Geometry: final body of the model. Coordinates: model frame, mm. A direction names the side the tool comes from. Give positions to 0.01 mm unless a question says otherwise; leave off trailing zeros. Loops run counter-clockwise (first coordinate to the right, second up) from the corner with the lowest first, then second, coordinate; pieces in that order, holes last.
Autodesk Inventor part; units mm, degrees
ref_plane "YZ Plane" through (0, 0, 0) normal (1, 0, 0) x (0, 1, 0)
ref_plane "XZ Plane" through (0, 0, 0) normal (0, 1, 0) x (-1, 0, 0)
ref_plane "XY Plane" through (0, 0, 0) normal (0, 0, 1) x (1, 0, 0)
sketch "Skizze1" plane through (0, 0, 0) normal (1, 0, 0) x (0, 1, 0)
  line L0 (105.1634, 173.9786) -> (55.1634, 173.9786)
  line L1 (55.1634, 173.9786) -> (55.1634, 93.4786)
  line L2 (55.1634, 93.4786) -> (105.1634, 93.4786)
  line L3 (105.1634, 93.4786) -> (105.1634, 173.9786)
  point P0 (0, 0)
  dimension "d0" = 80.5
  dimension "d1" = 50
extrude "Extrusion1" add sketch "Skizze1" along normal blind 5
sketch "Skizze2" plane through (5, 0, 0) normal (1, 0, 0) x (0, 0, -1)
  line L0 (-173.9786, 105.1639) -> (-168.9786, 105.1634)
  line L1 (-93.4786, 105.1634) -> (-173.9786, 105.1634)
  line L2 (-173.9786, 55.1634) -> (-93.4786, 55.1634)
  line L3 (-168.9786, 55.1634) -> (-173.9786, 55.1634)
  line L4 (-173.9786, 55.1634) -> (-173.9786, 105.1639)
  line L5 (-168.9786, 105.1634) -> (-168.9786, 55.1634)
  line L6 (-93.4786, 105.1634) -> (-98.4786, 105.1634)
  line L7 (-98.4786, 55.1634) -> (-93.4786, 55.1634)
  line L8 (-93.4786, 55.1634) -> (-93.4786, 105.1634)
  line L9 (-93.4786, 105.1634) -> (-98.4786, 105.1634)
  line L10 (-98.4786, 55.1634) -> (-98.4786, 105.1634)
  line L11 (-98.4786, 105.1634) -> (-93.4786, 105.1634)
  line L12 (-93.4786, 55.1634) -> (-98.4786, 55.1634)
  line L13 (-98.4786, 105.1634) -> (-93.4786, 105.1634)
  line L14 (-93.4786, 55.1634) -> (-98.4786, 55.1634)
  line L15 (-98.4786, 105.1634) -> (-93.4786, 105.1634)
  point P0 (0, 0)
  dimension "d4" = 5
  dimension "d5" = 5
extrude "Extrusion2" add sketch "Skizze2" along normal blind 70 contours L1 L8 L2 L10
sketch "Skizze3" plane through (5, 55.1634, 98.4786) normal (0, 0, 1) x (1, 0, 0)
  line L0 (22.2218, 34.8995) -> (57.5772, -0.4558)
  line L1 (57.5772, -0.4558) -> (56.5165, -1.5165)
  line L2 (56.5165, -1.5165) -> (21.1612, 33.8388)
  line L3 (21.1612, 33.8388) -> (22.2218, 34.8995)
  line L4 (-5, 50) -> (-5, 0)
  line L5 (21.1612, 33.8388) -> (38.8388, 16.1612)
  line L6 (0, 50) -> (70, 50)
  line L7 (57.5772, -0.4558) -> (56.5165, -1.5165)
  line L8 (56.5165, -1.5165) -> (57.5772, -0.4558)
  line L9 (51.6127, 5.5086) -> (50.5521, 4.4479)
  line L10 (50.5521, 4.4479) -> (56.5165, -1.5165)
  line L11 (57.5772, -0.4558) -> (51.6127, 5.5086)
  point P0 (-5, -55.1634)
  dimension "d8" = 1.5
  dimension "d9" = 50
  dimension "d10" = 45
  dimension "d35" = 16.1612
  dimension "d36" = 26.1612
sketch "Skizze4" plane through (0, 105.1634, 173.9786) normal (0, 1, 0) x (1, 0, 0)
  point P0 (0, 173.9786)
extrude "Extrusion3" cut sketch "Skizze3" against normal blind 3
sketch "Skizze5" plane through (5, 0, 0) normal (1, 0, 0) x (0, 0, -1)
  line L0 (-173.9786, 105.1634) -> (-173.9786, 55.1634)
  line L1 (-173.9786, 55.1634) -> (-168.9786, 55.1634)
  line L2 (-173.9786, 55.1634) -> (-98.4786, 55.1634)
  line L3 (-98.4786, 105.1634) -> (-173.9786, 105.1634)
  line L4 (-168.9786, 105.1634) -> (-173.9786, 105.1634)
  line L5 (-173.9786, 105.1634) -> (-173.9786, 55.1634)
  line L6 (-168.9786, 55.1634) -> (-168.9786, 105.1634)
  point P0 (0, 0)
  dimension "d15" = 5
extrude "Extrusion4" add sketch "Skizze5" along normal blind 70
sketch "Skizze6" plane through (5, 55.1634, 168.9786) normal (0, 0, -1) x (-1, 0, 0)
  line L0 (-57.5772, -0.4558) -> (-56.5165, -1.5165)
  line L1 (-56.5165, -1.5165) -> (-21.1612, 33.8388)
  line L2 (-21.1612, 33.8388) -> (-22.2218, 34.8995)
  line L3 (-22.2218, 34.8995) -> (-57.5772, -0.4558)
  line L4 (0, 50) -> (0, 0)
  line L5 (-21.1612, 33.8388) -> (-38.8388, 16.1612)
  line L6 (0, 0) -> (-70, 0)
  line L7 (-56.5165, -1.5165) -> (-57.5772, -0.4558)
  line L8 (-53.774, 3.3474) -> (-52.7133, 2.2867)
  line L9 (-52.7133, 2.2867) -> (-56.5165, -1.5165)
  line L10 (-57.5772, -0.4558) -> (-53.774, 3.3474)
  line L11 (0, 50) -> (-70, 50)
  point P0 (5, -55.1634)
  dimension "d18" = 1.5
  dimension "d19" = 50
  dimension "d20" = 45
  dimension "d22" = 1.5
  dimension "d37" = 21.1612
  dimension "d38" = 16.1612
extrude "Extrusion5" cut sketch "Skizze6" against normal blind 3
sketch "Skizze7" plane through (75, 0, 0) normal (1, 0, 0) x (0, 0, -1)
  point P0 (0, 0)
sketch "Skizze8" plane through (75, 0, 0) normal (1, 0, 0) x (0, 0, -1)
  point P0 (0, 0)
sketch "Skizze9" plane through (0, 0, 0) normal (-1, 0, 0) x (0, 0, 1)
  line L0 (93.4786, 55.1634) -> (93.4786, 105.1634)
  line L1 (93.4786, 105.1634) -> (173.9786, 105.1634)
  point P0 (0, 0)
  point P1 (133.7286, 80.1634)
  dimension "d26" = 40.25
  dimension "d27" = 25
hole "Bohrung1" at (0, 80.1634, 133.7286) direction (1, 0, 0) diameter 5 end through all
sketch "Skizze10" plane through (5, 55.1634, 98.4786) normal (0, 0, 1) x (1, 0, 0)
  point P0 (-5, -55.1634)
sketch "Skizze11" plane through (75, 0, 0) normal (1, 0, 0) x (0, 0, -1)
  point P0 (0, 0)
sketch "Skizze12" plane through (0, 55.1634, 173.9786) normal (0, 0, 1) x (1, 0, 0)
  line L0 (75, 50) -> (75, 0)
  circle A0 centre (75, 25) radius 5
  point P0 (0, -55.1634)
  dimension "d39" = 10
extrude "Extrusion6" cut sketch "Skizze12" against normal through all
sketch "Skizze13" plane through (0, 55.1634, 93.4786) normal (0, 0, -1) x (-1, 0, 0)
  line L0 (-75, 30) -> (-75, 50)
  line L1 (-62.1213, 0) -> (-75, 0)
  line L2 (-75, 50) -> (-65, 50)
  line L3 (-65, 50) -> (-65, 0)
  line L4 (-65, 0) -> (-75, 0)
  arc A0 (-75, 20) -> (-75, 30) centre (-75, 25) ccw
  line L5 (-75, 0) -> (-75, 20)
  line L6 (-75, 30) -> (-75, 50)
  point P0 (0, -55.1634)
  dimension "d42" = 10
extrude "Extrusion7" add sketch "Skizze13" along normal blind 3
sketch "Skizze14" plane through (0, 55.1634, 173.9786) normal (0, 0, 1) x (1, 0, 0)
  line L0 (62.1213, 0) -> (75, 0)
  line L1 (5, 50) -> (75, 50)
  line L2 (75, 0) -> (65, 0)
  line L3 (65, 0) -> (65, 50)
  line L4 (65, 50) -> (75, 50)
  arc A0 (75, 30) -> (75, 20) centre (75, 25) ccw
  arc A1 (75, 30) -> (75, 20) centre (75, 25) ccw
  line L5 (75, 50) -> (75, 30)
  line L6 (75, 20) -> (75, 0)
  point P0 (0, -55.1634)
  dimension "d45" = 10
extrude "Extrusion8" add sketch "Skizze14" along normal blind 3
sketch "Skizze15" plane through (75, 0, 0) normal (1, 0, 0) x (0, 0, -1)
  line L0 (-176.9786, 55.1634) -> (-176.9786, 75.1634)
  line L1 (-176.9786, 85.1634) -> (-176.9786, 105.1634)
  line L2 (-168.9786, 75.1634) -> (-176.9786, 75.1634)
  point P0 (0, 0)
  point P1 (-172.9786, 67.6634)
  point P2 (-172.9786, 92.6634)
  dimension "d48" = 4
  dimension "d49" = 4
  dimension "d50" = 25
  dimension "d51" = 7.5
sketch "Skizze16" plane through (75, 0, 0) normal (1, 0, 0) x (0, 0, -1)
  line L0 (-90.4786, 105.1634) -> (-90.4786, 85.1634)
  line L1 (-90.4786, 75.1634) -> (-90.4786, 55.1634)
  line L2 (-90.4786, 75.1634) -> (-98.4786, 75.1634)
  point P0 (0, 0)
  point P1 (-94.4786, 67.6634)
  point P2 (-94.4786, 92.6634)
  dimension "d52" = 25
  dimension "d53" = 4
  dimension "d54" = 4
  dimension "d55" = 7.5
sketch "Skizze17" plane through (75, 0, 0) normal (1, 0, 0) x (0, 0, -1)
  point P0 (0, 0)
hole "Bohrung2" at (75, 92.6634, 94.4786) at (75, 67.6634, 94.4786) direction (-1, 0, 0) diameter 2.75 depth 8 tip angle 118
hole "Bohrung3" at (75, 67.6634, 172.9786) at (75, 92.6634, 172.9786) direction (-1, 0, 0) diameter 2.75 depth 8 tip angle 118
properties part number "Spiegelhalter Objekthalter 1"
Item 1: Section query D-D on z = 153. Return loops of the section in (x, y), plus the area to 3 significant figures.
Values follow:
outline: (0, 55.16) - (5, 55.16) - (5, 105.16) - (0, 105.16) - close
area: 250 mm2
Item 2: Set-up query: faces 3 (the face through (70.94, 91.73, 95.49)), 4 (the face through (70, 80.3, 94.5)), 5 (the face through (32, 80, 93.479)), 6 (the face through (5, 85, 134)), 7 (the face through (44.427, 72.857, 170.458)). Return all of +Z, -Z, +X, -X, +Y, -Y with unobstructed straight access to the full face (end or side cutting, diameter ignored); none if empty.
Values follow:
face 3: +X
face 4: +Z, -Z, +X
face 5: -Z, -X, +Y, -Y
face 6: +X, +Y, -Y
face 7: none
Item 3: Draft query along Y for faces 1 (the face through (2.535, 82.604, 133.187)), 2 (the face through (0, 85, 134)). Return one class per face: +Y half, -Y half, draft (parallel to the pull), parting line (faces both ways), or undercut.
Values follow:
face 1: undercut
face 2: draft
Item 4: Ray query, probe 1 along Z at (x, y) = (72.5, 63); probe 2 along Z at (x, y) = (57, 80.5); probe 3 along X at (y, z) = (81.5, 136). Return the intervals inside material, ascending.
Values follow:
probe 1: z = 90.48 to 98.48, 168.98 to 176.98
probe 2: z = 93.48 to 98.48, 168.98 to 173.98
probe 3: x = 0 to 5
Item 5: Section query A-A on x = 15.5. Return loops of the section in (y, z), plus the area to 3 significant figures.
Values follow:
outline: (55.16, 93.48) - (105.16, 93.48) - (105.16, 98.48) - (55.16, 98.48) - close; (55.16, 168.98) - (105.16, 168.98) - (105.16, 173.98) - (55.16, 173.98) - close
area: 500 mm2
Item 6: Section query B-B on y = 61.5. Return loops of the section in (x, z).
Values follow:
outline: (0, 93.48) - (65, 93.48) - (65, 90.48) - (75, 90.48) - (75, 98.48) - (55.78, 98.48) - (55.78, 95.48) - (53.66, 95.48) - (53.66, 98.48) - (5, 98.48) - (5, 168.98) - (53.66, 168.98) - (53.66, 171.98) - (55.78, 171.98) - (55.78, 168.98) - (75, 168.98) - (75, 176.98) - (65, 176.98) - (65, 173.98) - (0, 173.98) - close
Item 7: Pin query (flat end, axial travel): pin 1 (8 mm diameter, centred on x = 55.5, z = 164.5, fed in from -Y); pin 2 (15 mm diameter, centred on x = 26, y = 74, fed in from -Z); pin 3 (2 mm diameter, centred on y = 67.66, z = 172.98, fed in from +X); pin 4 (8 mm diameter, centred on y = 80.16, z = 133.73, fed in from +X). Return the tip coordinate at first contact, or that it passes through.
Values follow:
pin 1: passes through
pin 2: stops at z = 93.48
pin 3: stops at x = 66.78
pin 4: stops at x = 5
Item 8: Section query C-C on x = 58. Return loops of the section in (y, z).
Values follow:
outline: (55.16, 93.48) - (105.16, 93.48) - (105.16, 98.48) - (59.28, 98.48) - (59.28, 95.48) - (57.16, 95.48) - (57.16, 98.48) - (55.16, 98.48) - close; (55.16, 168.98) - (57.16, 168.98) - (57.16, 171.98) - (59.28, 171.98) - (59.28, 168.98) - (105.16, 168.98) - (105.16, 173.98) - (55.16, 173.98) - close
